The listing builds one solid part. Answer for the finished solid, in the listing's coordinates (mm). A direction names the side the tool comes from. Round coordinates to 2 decimals unless told otherwise and drop trailing zeros. Loops run counter-clockwise (first coordinate to the right, second up) from the corner with the lowest first, then second, coordinate; pieces in that order, holes last. Notation, with made-up numbers: (86, 29) -> (136, 29) arc R18 cw to (136, 33) -> close; hole circle Ø5 at (3.5, 81). An arc over 180 degrees is marked (long way). Use a Markdown table: item, result. Add a question column.
Q1. Which of the six approach directions +Z, -Z, +X, -X, +Y, -Y give full straight-line access (tool end or side, diameter ignored) to faces 1 (the flat face through (-14, -2, 0)), 2 (the cylindrical face through (15.48, -1.5, 0.07)), 3 (the flat face through (0.196, 4.763, 2.859))?
Q2. Section D-D on y = -5.25 is taken. Give the vertices of the cut face in (x, z).
Q3. Section B-B on y = 0 is taken. Give the vertices of the cut face in (x, z).
Q4. Section C-C on z = -0.5 is taken. Give the vertices of the cut face in (x, y), then the cut area to 3 significant figures.
Q5. Section A-A on x = -1.5 is taken. Give the vertices of the cut face in (y, z).
Q6. Consider line 1 (X direction, y = 2, z = 3.25); line 2 (Z direction, x = 11, y = 5); line 3 (Z direction, x = -9.5, y = 1.25). Determine where each line is inside the solid, lowest interval first.
Q7. Given pin 1 Ø4 at (x, z) = (-12, 1) entering from -Y; pin 2 Ø3 at (x, z) = (2.5, -2.5) entering from -Y; pin 3 Ø6 at (x, y) = (4, 1.5) entering from +Z; pin 4 Ø2 at (x, y) = (-4, -1.5) entering from -Z, each flat-ended and moving along its own axis, determine where each tip first touches the part or whether it passes through.
from build123d import *

# Parameters (mm, degrees)
F1_DEPTH = 14
F2_R     = 1.5
F3_DEPTH = 3
F4_R     = 1.5
F5_DEPTH = 5


with BuildPart() as f1:
    # F0 (on Right) → F1 (new body, symmetric)
    with BuildSketch(Plane.YZ):
        Polygon((-3.3458015204, 5.4726269304), (-6.4123347074, -0.1612356475), (-3.0665331869, -5.6338625779), (3.3458015204, -5.4726269304), (6.4123347074, 0.1612356475), (3.0665331869, 5.6338625779), align=None)
    extrude(amount=F1_DEPTH, both=True)

    # F2 (on face) → F3 (join)
    with BuildSketch(Plane.YZ.offset(14)):
        Circle(F2_R)
    extrude(amount=F3_DEPTH)

    # F4 (on face) → F5 (join)
    with BuildSketch(Plane(origin=(-14, 0, 0), x_dir=(0, -1, 0), z_dir=(-1, 0, 0))):
        Circle(F4_R)
    extrude(amount=F5_DEPTH)


solid = f1.part
Checked values:
| question | item | result |
|---|---|---|
| 1 | face 1 | -X |
| 1 | face 2 | +X |
| 1 | face 3 | +Z, +X, -X, +Y |
| 2 | outline | (-14, -2.06) -> (14, -2.06) -> (14, 1.97) -> (-14, 1.97) -> close |
| 3 | outline | (-19, -1.5) -> (-14, -1.5) -> (-14, -5.56) -> (14, -5.56) -> (14, -1.5) -> (17, -1.5) -> (17, 1.5) -> (14, 1.5) -> (14, 5.56) -> (-14, 5.56) -> (-14, 1.5) -> (-19, 1.5) -> close |
| 4 | outline | (-19, -1.41) -> (-14, -1.41) -> (-14, -6.21) -> (14, -6.21) -> (14, -1.41) -> (17, -1.41) -> (17, 1.41) -> (14, 1.41) -> (14, 6.05) -> (-14, 6.05) -> (-14, 1.41) -> (-19, 1.41) -> close |
| 4 | area | 366 mm2 |
| 5 | outline | (-6.41, -0.16) -> (-3.07, -5.63) -> (3.35, -5.47) -> (6.41, 0.16) -> (3.07, 5.63) -> (-3.35, 5.47) -> close |
| 6 | line 1 | x = -14 to 14 |
| 6 | line 2 | z = -2.43 to 2.47 |
| 6 | line 3 | z = -5.53 to 5.59 |
| 7 | pin 1 | stops at y = -6.41 |
| 7 | pin 2 | stops at y = -5.9 |
| 7 | pin 3 | stops at z = 5.63 |
| 7 | pin 4 | stops at z = -5.62 |
